from build123d import *

# Parameters (mm, degrees)
F2_SIZE = 1.5
F3_R    = 1


with BuildPart() as f1:
    # F0 (on Front) → F1 (revolve)
    with BuildSketch(Plane.XZ):
        Polygon((15, 22), (15, 0), (24, 0), (24, 8), (19, 8), (19, 9), (24, 9), (24, 21.5), (22.5, 21.5), (22.5, 22), align=None)
    revolve(axis=Axis((0, 0, -3.522726), (0, 0, 1)))

    # F2
    f2_edges = [f1.edges().sort_by_distance(p)[0] for p in [
        (-24, 0, 0),
        (-15, 0, 0),
        (-15, 0, 22),
    ]]
    chamfer(f2_edges, length=F2_SIZE)

    # F3
    f3_edges = [f1.edges().sort_by_distance(p)[0] for p in [
        (-24, 0, 21.5),
    ]]
    fillet(f3_edges, radius=F3_R)


solid = f1.part
CAD build for the part. Positions are in the model's coordinates, mm. A direction names the side the tool comes from. Give positions to 0.01 mm unless a question says otherwise; leave off trailing zeros. Order: outer loops, then holes, each group sorted by start corner. A loop starts at its lowest first (then second) coordinate and runs counter-clockwise, first axis right, second up. Notation, with made-up numbers: (81, 53) -> (93, 53) arc R16 ccw to (93, 70) -> close; hole circle Ø6 at (85, 46). An arc over 180 degrees is marked (long way). Return JSON: item names as keys, results as strings.
Q1. Drill centre lines: line 1 (Y direction, x = 0, z = 15.5); line 2 (Z direction, x = -3.5, y = 20.5); line 3 (X direction, y = -0.5, z = 19.5). Where is each one in solid material? Low to high.
Working result:
{"line 1": "-24 to -15, 15 to 24", "line 2": "0 to 8, 9 to 22", "line 3": "-23.99 to -14.99, 14.99 to 23.99"}
Q2. Which spindle directions (+Z, -Z, +X, -X, +Y, -Y) get a long thin tool onto all of the face, cutting with end or side? Do faces 1 (the face through (17, -15, 21.5)), 2 (the face through (-23.977, 1.055, 4.796)), 3 (the face through (8.767, -16.856, 8.507)). Say none if no direction does.
Working result:
{"face 1": "+Z", "face 2": "+Z, -Z", "face 3": "none"}
Q3. Saw through at A-A (y = 0). Write the cut outline in (x, z).
Working result:
{"outline": "(-24, 1.5) -> (-22.5, 0) -> (-16.5, 0) -> (-15, 1.5) -> (-15, 20.5) -> (-16.5, 22) -> (-22.5, 22) -> (-22.5, 21.5) -> (-23, 21.5) arc R1 ccw to (-24, 20.5) -> (-24, 9) -> (-19, 9) -> (-19, 8) -> (-24, 8) -> close; (15, 1.5) -> (16.5, 0) -> (22.5, 0) -> (24, 1.5) -> (24, 8) -> (19, 8) -> (19, 9) -> (24, 9) -> (24, 20.5) arc R1 ccw to (23, 21.5) -> (22.5, 21.5) -> (22.5, 22) -> (16.5, 22) -> (15, 20.5) -> close"}
Q4. Saw through at C-C (z = 15.25). Write the cut outline in (x, y).
Working result:
{"outline": "circle Ø48 at (0, 0); hole circle Ø30 at (0, 0)"}
Q5. Mould opens along Y. For faces 4 (the face through (18, 7, 8)), 5 (the face through (-14.985, 0.66, 10.867)), 6 (the face through (10.382, -19.961, 21.754)) say: pulls with the +Y half, pulls with the -Y half, needs draft (parallel to the pull), parting line crosses it, or undercut.
Working result:
{"face 4": "needs draft", "face 5": "undercut", "face 6": "parting line crosses it"}
Q6. Flat gauge pins, fed straight in: pin 1 (3 mm diameter, centred on x = -11, z = 16.5, fed in from +Y); pin 2 (18 mm diameter, centred on x = 0, y = 0, fed in from +Z); pin 3 (5 mm diameter, centred on x = 16, z = 13.5, fed in from -Y); pin 4 (3 mm diameter, centred on x = -15, z = 4.5, fed in from +Y). Where does each tip first touch, or does it go through?
Working result:
{"pin 1": "y = 22.04", "pin 2": "through", "pin 3": "y = -19.84", "pin 4": "y = 19.84"}
